Could you check a few things on this model? Use its own coordinates, in mm. A direction names the side the tool comes from. Round coordinates to 2 decimals unless told otherwise and drop trailing zeros. Loops run counter-clockwise (first coordinate to the right, second up) from the corner with the lowest first, then second, coordinate; pieces in that order, holes last. Notation, with made-up numbers: M 56,15.25 L 110,15.25 A23 cw 110,53.25 Z; hole C 60.25,-26.75 d1. An arc over 180 degrees is marked long. Return JSON: item names as keys, results as strings. Group by question number.
```python
from build123d import *

# Parameters (mm, degrees)
FILLET047_R     = 7
SKETCH198_R     = 4.037815
SKETCH198_R_2   = 4.91935
POCKET063_DEPTH = 11.348059


with BuildPart() as part:
    # Sketch197 → Revolution001 (revolve)
    with BuildSketch(Plane.XZ):
        Polygon((0, 22.5), (36.347059, 22.5), (35.9, 42.5), (0, 42.5), align=None)
    revolve(axis=Axis((0, 0, 0), (0, 0, 1)))

    # Fillet047
    fillet047_edges = [part.edges().sort_by_distance(p)[0] for p in [
        (-35.9, 0, 42.5),
    ]]
    fillet(fillet047_edges, radius=FILLET047_R)

    # Sketch198 → Pocket063 (cut, through all)
    with BuildSketch(Plane.XZ.offset(25)):
        with Locations((-16.157519, 33.1)):
            Circle(SKETCH198_R)
        with Locations((16.157519, 33.1)):
            Circle(SKETCH198_R_2)
    extrude(amount=POCKET063_DEPTH, mode=Mode.SUBTRACT)


solid = part.part
```
1. On a 3-axis mill with a long thin cutter (end or side, diameter ignored), from which of +Z, -Z, +X, -X, +Y, -Y can I reach the whole of each face in a straight line? I mean faces 1 (the face through (0, 0, 42.5)), 2 (the face through (16, -25, 33)). Say none if no direction works.
2. If we section it at A-A, the plane z = 33.1: Please give me the cut outline in (x, y), then the cut area to 3 significant figures.
3. I need wall thicknesses on probe 1 along X at (y, z) = (-27, 33.1); probe 2 along X at (y, z) = (-28.5, 33.1); probe 3 along Z at (x, y) = (32.5, -14.5). Which ranges of each line are inside material? Lowest first, please.
4. If we section it at B-B, the plane x = 0: Please give me the cut outline in (y, z), then the cut area to 3 significant figures.
5. I'm going to push flat-ended pins straight in: pin 1 Ø5 at (y, z) = (16, 36.5) entering from +X; pin 2 Ø7.5 at (x, z) = (-16.16, 33.1) entering from +Y; pin 3 Ø9 at (x, z) = (-15, 32.5) entering from -Y. Where does each tip first touch, or does it pass through?
6. If we section it at D-D, the plane z = 40.5: Please give me the cut outline in (x, y).
7. We'd pull the mould along X, two halves only. Please class faces 3 (the face through (11.243, -28.561, 33.316)), 4 (the face through (1, 1, 22.5)), 5 (the face through (-4.71, 35.89, 29.17)): +X half, -X half, draft (parallel to the pull), parting line (faces both ways), or undercut.
Geometry results:
{
 "1": {"face 1": "+Z, +X, -X, +Y, -Y", "face 2": "-Y"},
 "2": {"outline": "M -20.2,-29.93 L -20.2,-25 L -12.12,-25 L -12.12,-34.02 A36.11 ccw 11.24,-34.32 L 11.24,-25 L 21.08,-25 L 21.08,-29.32 A36.11 ccw long Z", "area": "3,970 mm^2"},
 "3": {"probe 1": "-23.98 to -20.2, -12.12 to 11.24, 21.08 to 23.98", "probe 2": "-22.17 to -20.2, -12.12 to 11.24, 21.08 to 22.17", "probe 3": "22.5 to 38.01"},
 "4": {"outline": "M -36.35,22.5 L 36.35,22.5 L 36.05,35.66 A7 ccw 29.05,42.5 L -29.05,42.5 A7 ccw -36.05,35.66 Z", "area": "1,420 mm^2"},
 "5": {"pin 1": "x = 33.39", "pin 2": "y = 33.91", "pin 3": "y = -34.57"},
 "6": {"outline": "C 0,0 d67.91"},
 "7": {"face 3": "undercut", "face 4": "draft", "face 5": "parting line"}
}
